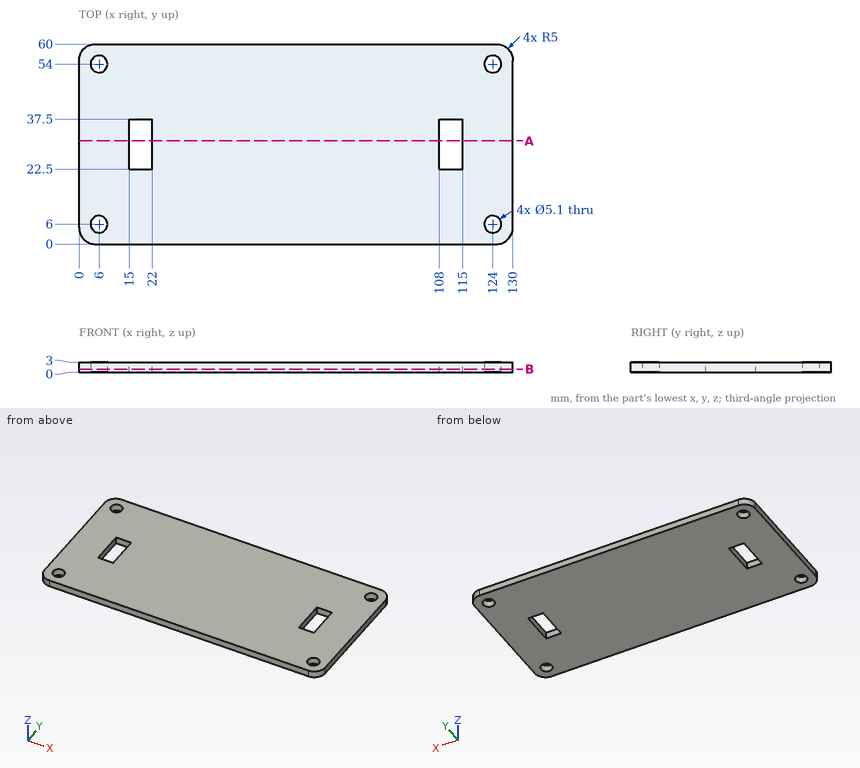
Input: dimensioned drawing with shaded views. Units: mm. Origin: part minimum x, y, z. Give positions to 0.01 mm unless a question says otherwise; leave off trailing zeros. Write each loop counter-clockwise with the first axis right and the second up, starting at its lowest first coordinate (ties: lowest second). Pieces come first, ordered by that corner, then holes. Notation, with made-up numbers: M 9,-12.75 L 37,-12.75 A15 cw 37,-5.75 Z; hole C -24,-21.75 d3. An arc over 180 degrees is marked long. Return JSON: item names as keys, results as strings. Group by question number.
1) Material intervals for line 1 along Y through (x, z) = (124, 1.45); line 2 along Y through (x, z) = (109.5, 0.9); line 3 along X through (y, z) = (23, 2.5), sorted ascending. Write a range as [from, to].
2) Cut plane B-B, the plane z = 0.9. Output: boundary loops of the cut face in (x, y).
3) Pin query (flat end, axial travel): P1, Ø4.5, axis at x = 124, y = 6, coming from the -Z side. Return the tip coordinate at first contact, or that it passes through.
4) Cut plane A-A, the plane y = 31. Output: boundary loops of the cut face in (x, z).
Recorded:
{
 "1": {"line 1": "y = [0, 3.45], [8.55, 51.45], [56.55, 60]", "line 2": "y = [0, 22.5], [37.5, 60]", "line 3": "x = [0, 15], [22, 108], [115, 130]"},
 "2": {"outline": "M 0,5 A5 ccw 5,0 L 125,0 A5 ccw 130,5 L 130,55 A5 ccw 125,60 L 5,60 A5 ccw 0,55 Z; hole C 6,6 d5.1; hole C 6,54 d5.1; hole M 15,22.5 L 22,22.5 L 22,37.5 L 15,37.5 Z; hole M 108,22.5 L 115,22.5 L 115,37.5 L 108,37.5 Z; hole C 124,6 d5.1; hole C 124,54 d5.1"},
 "3": {"P1": "passes through"},
 "4": {"outline": "M 0,0 L 15,0 L 15,3 L 0,3 Z; M 22,0 L 108,0 L 108,3 L 22,3 Z; M 115,0 L 130,0 L 130,3 L 115,3 Z"}
}
